CAD build for the part. Positions are in the model's coordinates, mm. A direction names the side the tool comes from. Give positions to 0.01 mm unless a question says otherwise; leave off trailing zeros. Order: outer loops, then holes, each group sorted by start corner. A loop starts at its lowest first (then second) coordinate and runs counter-clockwise, first axis right, second up.
Item 1: Flat gauge pin, fed straight in: P1, Ø1.5, axis at x = 3, z = 4, coming from the -Y side. Where does the tip first touch, or does it go through?
Item 2: Wall check: L1, parallel to Y at x = -0.5, z = 1.9; L2, parallel to Y at x = 0.5, z = 1.1; L3, parallel to X at y = -82.5, z = 0.7. Give the ranges that are in metal, low to high.
Item 3: Which spindle directions (+Z, -Z, +X, -X, +Y, -Y) get a long thin tool onto all of the face, cutting with end or side? Do faces 1 (the flat face through (3, -1, 2.5)), 2 (the flat face through (-5, -2, 1)). Say none if no direction does.
Item 4: Band-saw the part on A-A on y = 53. Give the cut face in (x, z).
```python
from build123d import *

# Parameters (mm, degrees)
F0_W           = 10
F0_H           = 320
F1_DEPTH       = 2.5
F0_H_2         = 10
F2_DEPTH       = 5
F3_T1_DEPTH    = 31.6506350946
F5_D           = 2.5
F5_DEPTH       = 2.5
F5_CSINK_D     = 5
F5_CSINK_ANGLE = 90
F5_TIP         = 0.7510757738


# Not quite as in the source:
# - a fillet or chamfer that OpenCascade refuses, or shapes differently, is made with other operations: its cross-section is extruded or revolved along the edge and cut away or added


with BuildPart() as f1:
    # F0 (on Top) → F1 (new body)
    with BuildSketch(Plane.XY):
        with Locations((0, -5)):
            Rectangle(F0_W, F0_H)
    extrude(amount=F1_DEPTH)

    # F0 (on Top) → F2 (join)
    with BuildSketch(Plane.XY):
        with Locations((0, 160)):
            Rectangle(F0_W, F0_H_2)
    extrude(amount=F2_DEPTH)

    # F3: fillet of radius 5 on 1 edges, made by hand

    # F3_s2 → F3_t1 (cut)
    with BuildSketch(Plane.YZ.offset(-15.8253175473)):
        with BuildLine():
            ThreePointArc((-160.6698729811, 2.5), (-163.1698729811, 1.8301270189), (-165, 0))
            Line((-165, 0), (-165, 2.5))
            Line((-165, 2.5), (-160.6698729811, 2.5))
        make_face()
    extrude(amount=F3_T1_DEPTH, mode=Mode.SUBTRACT)

    # F5
    with Locations(Plane.XY.offset(2.5)):
        with Locations((0, 82.5), (0, 0), (0.1304344232, -82.5)):
            CounterSinkHole(F5_D / 2, F5_CSINK_D / 2, depth=F5_DEPTH, counter_sink_angle=F5_CSINK_ANGLE)
            with Locations((0, 0, -(F5_DEPTH + F5_TIP / 2))):  # 118° drill point
                Cone(0, F5_D / 2, F5_TIP, mode=Mode.SUBTRACT)


solid = f1.part
```
The answers:
1. P1: stops at y = 155
2. L1: y = -163.04 to -84.29, -80.71 to -1.83, 1.83 to 80.67, 84.33 to 165
2. L2: y = -164.14 to -83.69, -81.31 to -1.15, 1.15 to 81.35, 83.65 to 165
2. L3: x = -5 to -1.12, 1.38 to 5
3. face 1: +Z, +X, -X, -Y
3. face 2: +Z, -Z, -X, +Y, -Y
4. outline: (-5, 0) - (5, 0) - (5, 2.5) - (-5, 2.5) - close
